The model under review builds one solid part; all positions refer to its coordinate system, in mm. A direction names the side the tool comes from. Give positions to 0.01 mm unless a question says otherwise; leave off trailing zeros. Order: outer loops, then holes, each group sorted by start corner. A loop starts at its lowest first (then second) coordinate and runs counter-clockwise, first axis right, second up.
```python
from build123d import *

# Parameters (mm, degrees)
SKETCH_1_R      = 1.1
EXTRUDE_1_DEPTH = 5
EXTRUDE_2_DEPTH = 5
FILLET_1_R      = 1.5


with BuildPart() as part:
    # ｽｹｯﾁ1 → ﾎﾞｽ - 押し出し1 (new body)
    with BuildSketch(Plane.XY):
        with BuildLine():
            Line((-5, 60), (5, 60))
            Line((5, 60), (5, 29.949874371))
            ThreePointArc((5, 29.949874371), (5.425728922, 27.063123025), (6.666666667, 24.422166387))
            ThreePointArc((6.666666667, 24.422166387), (8, 20), (6.666666667, 15.577833613))
            ThreePointArc((6.666666667, 15.577833613), (5.425728922, 12.936876975), (5, 10.050125629))
            Line((5, 10.050125629), (5, 0))
            Line((5, 0), (-5, 0))
            Line((-5, 0), (-5, 10.050125629))
            ThreePointArc((-5, 10.050125629), (-5.425728922, 12.936876975), (-6.666666667, 15.577833613))
            ThreePointArc((-6.666666667, 15.577833613), (-8, 20), (-6.666666667, 24.422166387))
            ThreePointArc((-6.666666667, 24.422166387), (-5.425728922, 27.063123025), (-5, 29.949874371))
            Line((-5, 29.949874371), (-5, 60))
        make_face()
        with Locations((0, 20)):
            Circle(SKETCH_1_R, mode=Mode.SUBTRACT)
        with Locations((0, 14)):
            Circle(SKETCH_1_R, mode=Mode.SUBTRACT)
        with Locations((-4.242640687, 15.757359313)):
            Circle(SKETCH_1_R, mode=Mode.SUBTRACT)
        with Locations((-6, 20)):
            Circle(SKETCH_1_R, mode=Mode.SUBTRACT)
        with Locations((-4.242640687, 24.242640687)):
            Circle(SKETCH_1_R, mode=Mode.SUBTRACT)
        with Locations((0, 26)):
            Circle(SKETCH_1_R, mode=Mode.SUBTRACT)
        with Locations((4.242640687, 24.242640687)):
            Circle(SKETCH_1_R, mode=Mode.SUBTRACT)
        with Locations((6, 20)):
            Circle(SKETCH_1_R, mode=Mode.SUBTRACT)
        with Locations((4.242640687, 15.757359313)):
            Circle(SKETCH_1_R, mode=Mode.SUBTRACT)
    extrude(amount=EXTRUDE_1_DEPTH)

    # ｽｹｯﾁ2 → ﾎﾞｽ - 押し出し2 (add)
    with BuildSketch(Plane(origin=(0, 0, 0), x_dir=(-1, 0, 0), z_dir=(0, 0, -1))):
        with BuildLine():
            Line((5, 10.050125629), (5, 0))
            Line((5, 0), (15, 0))
            ThreePointArc((15, 0), (13.531166576, 30.48861935), (21.328075812, 60))
            Line((21.328075812, 60), (5, 60))
            Line((5, 60), (5, 29.949874371))
            ThreePointArc((5, 29.949874371), (5.425728922, 27.063123025), (6.666666667, 24.422166387))
            ThreePointArc((6.666666667, 24.422166387), (8, 20), (6.666666667, 15.577833613))
            ThreePointArc((6.666666667, 15.577833613), (5.425728922, 12.936876975), (5, 10.050125629))
        make_face()
    extrude(amount=-EXTRUDE_2_DEPTH)

    # ﾌｨﾚｯﾄ1
    fillet_1_edges = [part.edges().sort_by_distance(p)[0] for p in [
        (5, 0, 2.5),
        (5, 60, 2.5),
        (-21.328075812, 60, 2.5),
        (-15, 0, 2.5),
    ]]
    fillet(fillet_1_edges, radius=FILLET_1_R)


solid = part.part
```
1. Take a section at A-A (x = 0). Write out the cut boundary in (y, z).
2. Insertion check: pin 1 (1 mm diameter, centred on y = 41, z = 4.5, fed in from +X). The pin has a flat end and moves straight along its axis. Give the tip position at first contact, or say it passes through.
3. To check wall thickness, follow line 1 (Y direction, x = 0, z = 3.35); line 2 (Y direction, x = 0.5, z = 4.7); line 3 (Y direction, x = -6.25, z = 1.9). State the ranges of each line that lie inside material, in increasing order.
4. Draft analysis for pull direction Y (two halves, no side actions). For faces 3 (the cylindrical face through (5.414, 27.102, 2.465)), 4 (the cylindrical face through (-4.481, 14.684, 2.465)), 5 (the flat face through (-6, 30, 5)), state which applies: pulls with the +Y half, pulls with the -Y half, needs draft (parallel to the pull), parting line crosses it, or undercut.
5. Take a section at C-C (x = 6). Write out the cut boundary in (y, z).
6. Take a section at D-D (z = 4.4). Count the separate pieces of the cut face and the enclosed holes in it, and give its area (3 significant figures).
7. Take a section at B-B (y = 20). Write out the cut boundary in (x, z), and give its area (3 significant figures).
8. For faces 1 (the flat face through (5, 6, 2)), 2 (the cylindrical face through (4.004, 14.684, 2.465)), list the 3-axis set-ups (+Z, -Z, +X, -X, +Y, -Y) from which the entire face can be reached by the end or side of a thin tool; tool diameter is ignored.
Answer:
1. outline: (0, 0) - (12.9, 0) - (12.9, 5) - (0, 5) - close; (15.1, 0) - (18.9, 0) - (18.9, 5) - (15.1, 5) - close; (21.1, 0) - (24.9, 0) - (24.9, 5) - (21.1, 5) - close; (27.1, 0) - (60, 0) - (60, 5) - (27.1, 5) - close
2. pin 1: stops at x = 5
3. line 1: y = 0 to 12.9, 15.1 to 18.9, 21.1 to 24.9, 27.1 to 60
3. line 2: y = 0 to 13.02, 14.98 to 19.02, 20.98 to 25.02, 26.98 to 60
3. line 3: y = 0 to 18.93, 21.07 to 60
4. face 3: pulls with the +Y half
4. face 4: undercut
4. face 5: needs draft
5. outline: (14.41, 0) - (18.9, 0) - (18.9, 5) - (14.41, 5) - close; (21.1, 0) - (25.59, 0) - (25.59, 5) - (21.1, 5) - close
6. separate pieces: 1
6. enclosed holes: 9
6. area: 1,190 mm2
7. outline: (-12.98, 0) - (-7.1, 0) - (-7.1, 5) - (-12.98, 5) - close; (-4.9, 0) - (-1.1, 0) - (-1.1, 5) - (-4.9, 5) - close; (1.1, 0) - (4.9, 0) - (4.9, 5) - (1.1, 5) - close; (7.1, 0) - (8, 0) - (8, 5) - (7.1, 5) - close
7. area: 71.9 mm2
8. face 1: +Z, -Z, +X, -Y
8. face 2: +Z, -Z
